Source: CAD feature listing. Evaluate the final solid. Frame: model axes, mm. A direction names the side the tool comes from. Give positions to 0.01 mm unless a question says otherwise; leave off trailing zeros. Order: outer loops, then holes, each group sorted by start corner. A loop starts at its lowest first (then second) coordinate and runs counter-clockwise, first axis right, second up. Notation, with made-up numbers: (-9, 48) - (33, 48) arc R21 ccw to (33, 59) - close; hole circle Ø8 at (71.25, -12.5). An arc over 180 degrees is marked (long way). Use CSV: the item, a comma, the result in double quotes.
```python
from build123d import *

# Parameters (mm, degrees)
PAD_DEPTH    = 1.5
SKETCH001_R  = 4.85
PAD001_DEPTH = 8.8
SKETCH002_W  = 0.5
SKETCH002_H  = 0.5
PAD002_DEPTH = 26
SKETCH003_W  = 0.5
SKETCH003_H  = 0.5
PAD003_DEPTH = 24.5


with BuildPart() as part:
    # Sketch → Pad (new body)
    with BuildSketch(Plane.XY):
        with BuildLine():
            ThreePointArc((4.906655, 1.867414), (-5.25, 0), (4.906655, -1.867414))
            Line((4.906655, -1.867414), (4.906655, 1.867414))
        make_face()
    extrude(amount=PAD_DEPTH)

    # Sketch001 (on Face3 of Pad) → Pad001 (join)
    with BuildSketch(Plane(origin=(0, 0, 0), x_dir=(1, 0, 0), z_dir=(0, 0, -1))):
        Circle(SKETCH001_R)
    extrude(amount=PAD001_DEPTH)

    # Sketch002 (on Face4 of Pad001) → Pad002 (join)
    with BuildSketch(Plane.XY.offset(1.5)):
        with Locations((-1.27, 0)):
            Rectangle(SKETCH002_W, SKETCH002_H)
    extrude(amount=PAD002_DEPTH)

    # Sketch003 (on Face4 of Pad001) → Pad003 (join)
    with BuildSketch(Plane.XY.offset(1.5)):
        with Locations((1.27, 0)):
            Rectangle(SKETCH003_W, SKETCH003_H)
    extrude(amount=PAD003_DEPTH)


solid = part.part
```
Item 1: Section D-D on z = -0.5. Return the cut outline in (x, y), then the cut area to 3 significant figures.
Filled in:
outline,"circle Ø9.7 at (0, 0)"
area,"73.9 mm2"
Item 2: Section A-A on z = 12.5. Return the cut outline in (x, y), then the cut area to 3 significant figures.
Filled in:
outline,"(-1.52, -0.25) - (-1.02, -0.25) - (-1.02, 0.25) - (-1.52, 0.25) - close; (1.02, -0.25) - (1.52, -0.25) - (1.52, 0.25) - (1.02, 0.25) - close"
area,"0.500 mm2"
Item 3: Set-up query: faces 1 (the flat face through (-5, 1, 0)), 2 (the cylindrical face through (-5.246, 0.204, 0.74)). Return all of +Z, -Z, +X, -X, +Y, -Y with unobstructed straight access to the full face (end or side cutting, diameter ignored); none if empty.
Filled in:
face 1,"-Z"
face 2,"+Z, -Z"
Item 4: Section B-B on y = 4.5. Return the cut outline in (x, z).
Filled in:
outline,"(-2.7, 0) - (-1.81, 0) - (-1.81, -8.8) - (1.81, -8.8) - (1.81, 0) - (2.7, 0) - (2.7, 1.5) - (-2.7, 1.5) - close"
Item 5: Section C-C on x = 0. Return the cut outline in (y, z).
Filled in:
outline,"(-5.25, 0) - (-4.85, 0) - (-4.85, -8.8) - (4.85, -8.8) - (4.85, 0) - (5.25, 0) - (5.25, 1.5) - (-5.25, 1.5) - close"
Item 6: First-contact query: pin 1 (1.5 mm diameter, centred on y = -0.5, z = 11.5, fed in from +X); pin 2 (5 mm diameter, centred on x = -0.5, y = 2.5, fed in from +Z); pin 3 (4 mm diameter, centred on x = 0.5, z = 16.5, fed in from +Y); pin 4 (1 mm diameter, centred on x = 0, y = 1.5, fed in from +Z). Flat tips, straight axial feed; report the tip coordinate or a pass-through.
Filled in:
pin 1,"stops at x = 1.52"
pin 2,"stops at z = 27.5"
pin 3,"stops at y = 0.25"
pin 4,"stops at z = 1.5"
Item 7: Material intervals for line 1 (Z direction, x = -1.5, y = 4); line 2 (Y direction, x = 1.25, z = 10); line 3 (Y direction, x = -0.25, z = -3.5), sorted ascending. Write a range as from..to.
Filled in:
line 1,"z = -8.8..1.5"
line 2,"y = -0.25..0.25"
line 3,"y = -4.84..4.84"
